Geometry: see drawing. Coordinates: mm, zero at the bounding-box minimum. Coordinates: 2 decimals unless noted, no trailing zeros. Loops run counter-clockwise (first coordinate to the right, second up) from the corner with the lowest first, then second, coordinate; pieces in that order, holes last. Notation, with made-up numbers: (-5.75, -23.75) - (25.25, -23.75) arc R27 cw to (25.25, 2.25) - close; hole circle Ø11 at (-24, 42). An arc over 180 degrees is marked (long way). Answer in a Markdown table with one row per item.
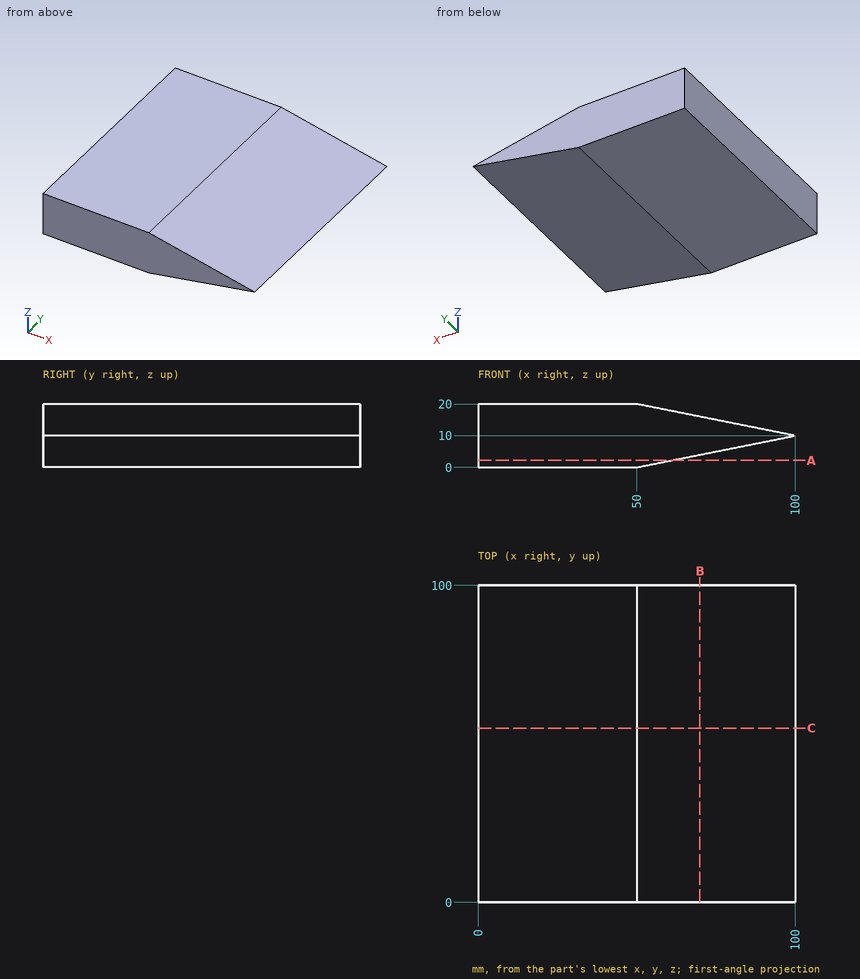
(1) Ray query, probe 1 along Z at (x, y) = (89, 76). Return the intervals inside material, ascending.
Verdict:
| item | result |
|---|---|
| probe 1 | z = 7.8 to 12.2 |
(2) Cut plane C-C on y = 55. Output: boundary loops of the cut face in (x, z).
Verdict:
| item | result |
|---|---|
| outline | (0, 0) - (50, 0) - (100, 10) - (50, 20) - (0, 20) - close |
(3) First-contact query: pin 1 Ø10 at (x, y) = (61.5, 12) entering from +Z; pin 2 Ø10 at (x, y) = (60.5, 51) entering from +Z; pin 3 Ø10 at (x, y) = (63, 28.5) entering from -Z. Flat tips, straight axial feed; report the tip coordinate or a pass-through.
Verdict:
| item | result |
|---|---|
| pin 1 | stops at z = 18.7 |
| pin 2 | stops at z = 18.9 |
| pin 3 | stops at z = 1.6 |
(4) Cut plane B-B on x = 70. Output: boundary loops of the cut face in (y, z), then the cut area to 3 significant figures.
Verdict:
| item | result |
|---|---|
| outline | (0, 4) - (100, 4) - (100, 16) - (0, 16) - close |
| area | 1,200 mm² |
(5) Cut plane A-A on z = 2.25. Output: boundary loops of the cut face in (x, y).
Verdict:
| item | result |
|---|---|
| outline | (0, 0) - (61.25, 0) - (61.25, 100) - (0, 100) - close |
